For this review, take the finished solid that the model builds, in its own axes (mm). A direction names the side the tool comes from. Give positions to 0.01 mm unless a question says otherwise; leave off trailing zeros. Write each loop counter-clockwise with the first axis right and the second up, starting at its lowest first coordinate (ties: lowest second). Pieces come first, ordered by that corner, then holes. Notation, with made-up numbers: (-15, 51.25) -> (-4, 51.25) arc R24 cw to (-4, 70.25) -> close; hole circle Ø9 at (59, -31). An arc over 180 degrees is marked (long way). Return JSON: item names as keys, results as strings.
from build123d import *

# Parameters (mm, degrees)
SKETCH_1_W          = 45.4
SKETCH_1_H          = 35
SKETCH_1_R          = 1.65
EXTRUDE_1_DEPTH     = 10
FILLET_1_R          = 2
SKETCH_2_R          = 1.65
CUT_EXTRUDE_1_DEPTH = 10


with BuildPart() as part:
    # ｽｹｯﾁ1 → ﾎﾞｽ - 押し出し1 (new body)
    with BuildSketch(Plane.XY):
        with Locations((22.7, 17.5)):
            Rectangle(SKETCH_1_W, SKETCH_1_H)
        with Locations((10, 5)):
            Circle(SKETCH_1_R, mode=Mode.SUBTRACT)
        with Locations((35.4, 5)):
            Circle(SKETCH_1_R, mode=Mode.SUBTRACT)
        with Locations((5, 30)):
            Circle(SKETCH_1_R, mode=Mode.SUBTRACT)
        with Locations((30.4, 30)):
            Circle(SKETCH_1_R, mode=Mode.SUBTRACT)
    extrude(amount=EXTRUDE_1_DEPTH)

    # ﾌｨﾚｯﾄ1
    fillet_1_edges = [part.edges().sort_by_distance(p)[0] for p in [
        (0, 35, 5),
        (45.4, 35, 5),
        (45.4, 0, 5),
        (0, 0, 5),
    ]]
    fillet(fillet_1_edges, radius=FILLET_1_R)

    # ｽｹｯﾁ2 → ｶｯﾄ - 押し出し1 (cut)
    with BuildSketch(Plane.XZ):
        with Locations(Location((2.7, 5, 0), (0, 0, 270))):
            Circle(SKETCH_2_R)
        with Locations(Location((42.7, 5, 0), (0, 0, 270))):
            Circle(SKETCH_2_R)
    extrude(amount=-CUT_EXTRUDE_1_DEPTH, mode=Mode.SUBTRACT)


solid = part.part
1. Add section C-C, the plane z = 1. State the section outline as (x, y) points.
Results found:
{"outline": "(0, 2) arc R2 ccw to (2, 0) -> (43.4, 0) arc R2 ccw to (45.4, 2) -> (45.4, 33) arc R2 ccw to (43.4, 35) -> (2, 35) arc R2 ccw to (0, 33) -> close; hole circle Ø3.3 at (5, 30); hole circle Ø3.3 at (10, 5); hole circle Ø3.3 at (30.4, 30); hole circle Ø3.3 at (35.4, 5)"}
2. For pin 1 (3 mm diameter, centred on x = 2.7, z = 5, fed in from -Y), flat-tipped, find the tip position at first contact; note if it passes through.
Results found:
{"pin 1": "stops at y = 10"}
3. For faces 1 (the flat face through (22, 35, 5)), 2 (the cylindrical face through (43.815, 4.93, 6.216)), list the 3-axis set-ups (+Z, -Z, +X, -X, +Y, -Y) from which the entire face can be reached by the end or side of a thin tool; tool diameter is ignored.
Results found:
{"face 1": "+Z, -Z, +X, -X, +Y", "face 2": "-Y"}
4. Add section D-D, the plane x = 35.4. State the section outline as (y, z) points, plus the area to 3 significant figures.
Results found:
{"outline": "(0, 0) -> (3.35, 0) -> (3.35, 10) -> (0, 10) -> close; (6.65, 0) -> (35, 0) -> (35, 10) -> (6.65, 10) -> close", "area": "317 mm²"}
5. Add section B-B, the plane y = 30. State the section outline as (x, z) points.
Results found:
{"outline": "(0, 0) -> (3.35, 0) -> (3.35, 10) -> (0, 10) -> close; (6.65, 0) -> (28.75, 0) -> (28.75, 10) -> (6.65, 10) -> close; (32.05, 0) -> (45.4, 0) -> (45.4, 10) -> (32.05, 10) -> close"}
6. The part is to be moulded in two halves that separate along X. For faces 3 (the flat face through (22, 0, 5)), 4 (the cylindrical face through (33.75, 5.07, 4.93)), 5 (the cylindrical face through (44.8, 34.43, 5.07)), 6 (the flat face through (3, 10, 5)), say which applies: +X half, -X half, draft (parallel to the pull), parting line (faces both ways), or undercut.
Results found:
{"face 3": "draft", "face 4": "undercut", "face 5": "+X half", "face 6": "undercut"}
7. Add section A-A, the plane y = 5. State the section outline as (x, z) points.
Results found:
{"outline": "(0, 0) -> (8.35, 0) -> (8.35, 10) -> (0, 10) -> close; (11.65, 0) -> (33.75, 0) -> (33.75, 10) -> (11.65, 10) -> close; (37.05, 0) -> (45.4, 0) -> (45.4, 10) -> (37.05, 10) -> close; hole circle Ø3.3 at (2.7, 5); hole circle Ø3.3 at (42.7, 5)"}
8. To check wall thickness, follow probe 1 along X at (y, z) = (5.5, 3.25); probe 2 along Y at (x, z) = (5, 4); probe 3 along Y at (x, z) = (35.4, 4). State the ranges of each line that lie inside material, in increasing order.
Results found:
{"probe 1": "x = 0 to 8.43, 11.57 to 33.83, 36.97 to 45.4", "probe 2": "y = 0 to 28.35, 31.65 to 35", "probe 3": "y = 0 to 3.35, 6.65 to 35"}
